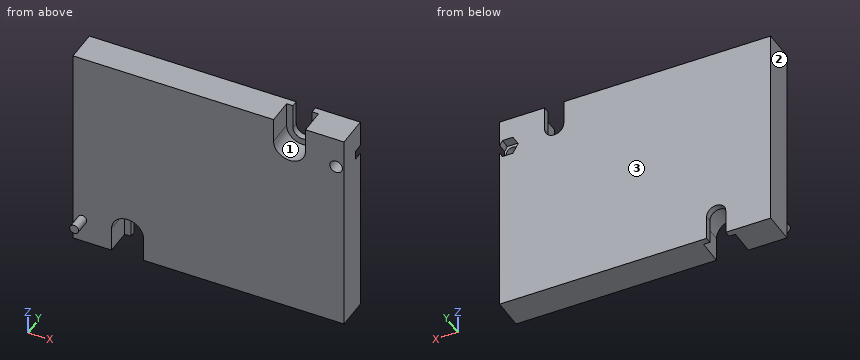
Autodesk Inventor part; units mm, degrees
ref_plane "YZ Plane" through (0, 0, 0) normal (1, 0, 0) x (0, 1, 0)
ref_plane "XZ Plane" through (0, 0, 0) normal (0, 1, 0) x (-1, 0, 0)
ref_plane "XY Plane" through (0, 0, 0) normal (0, 0, 1) x (1, 0, 0)
sketch "Sketch1" plane through (0, 0, 0) normal (0, 1, 0) x (-1, 0, 0)
  line L0 (42.5, -32.5) -> (42.5, 32.5)
  line L1 (-42.5, 32.5) -> (-42.5, -32.5)
  line L2 (-42.5, -32.5) -> (42.5, 32.5) construction
  line L3 (42.5, -32.5) -> (-42.5, 32.5) construction
  line L4 (-25.4, -24.765) -> (25.4, -24.765) construction
  line L5 (25.4, -24.765) -> (25.4, 24.765) construction
  line L6 (25.4, 24.765) -> (-25.4, 24.765) construction
  line L7 (-25.4, 24.765) -> (-25.4, -24.765) construction
  line L8 (-25.4, -24.765) -> (25.4, 24.765) construction
  line L9 (25.4, -24.765) -> (-25.4, 24.765) construction
  arc A0 (-28.4, 24.765) -> (-22.4, 24.765) centre (-25.4, 24.765) ccw
  arc A1 (-30.4, 24.765) -> (-20.4, 24.765) centre (-25.4, 24.765) ccw
  arc A2 (28.4, -24.765) -> (22.4, -24.765) centre (25.4, -24.765) ccw
  arc A3 (30.4, -24.765) -> (20.4, -24.765) centre (25.4, -24.765) ccw
  line L10 (-20.4, 32.5) -> (-20.4, 24.765)
  line L11 (-30.4, 32.5) -> (-30.4, 24.765)
  line L12 (-28.4, 32.5) -> (-28.4, 24.765)
  line L13 (-22.4, 32.5) -> (-22.4, 24.765)
  line L14 (30.4, -24.765) -> (30.4, -32.5)
  line L15 (28.4, -24.765) -> (28.4, -32.5)
  line L16 (22.4, -24.765) -> (22.4, -32.5)
  line L17 (20.4, -24.765) -> (20.4, -32.5)
  line L18 (-42.5, -32.5) -> (22.4, -32.5)
  line L19 (28.4, -32.5) -> (42.5, -32.5)
  line L20 (42.5, 32.5) -> (-22.4, 32.5)
  line L21 (-28.4, 32.5) -> (-42.5, 32.5)
  point P0 (0, 0)
  dimension "d2" = 50.8
  dimension "d3" = 49.53
  dimension "d4" = 6
  dimension "d5" = 10
sketch "Sketch2" plane through (0, 0, 0) normal (0, 1, 0) x (-1, 0, 0)
  line L0 (-43, -29.25) -> (43, -29.25)
  line L1 (43, -29.25) -> (43, 29.25)
  line L2 (43, 29.25) -> (-43, 29.25)
  line L3 (-43, 29.25) -> (-43, -29.25)
  line L4 (-43, -29.25) -> (43, 29.25) construction
  line L5 (43, -29.25) -> (-43, 29.25) construction
  circle A0 centre (39.6, -24.85) radius 1.4
  line L6 (41, -24.85) -> (39.6, -24.85)
  line L7 (39.6, -24.85) -> (39.6, -26.25)
  circle A1 centre (-40, 22.75) radius 2
  line L8 (-38, 22.75) -> (-43, 22.75) construction
  line L9 (-40, 24.75) -> (-40, 29.25) construction
  line L10 (-40, 24.75) -> (-40, 22.75) construction
  point P0 (0, 0)
  dimension "d6" = 86
  dimension "d7" = 58.5
  dimension "d8" = 2.8
  dimension "d9" = 3
  dimension "d10" = 2
  dimension "d11" = 4
  dimension "d12" = 5
  dimension "d13" = 4.5
extrude "Extrusion1" add sketch "Sketch1" along normal blind 10
extrude "Extrusion2" cut sketch "Sketch1" along normal blind 8 contours L19 L15 A2 L16 L18 L17 A3 L14 | L10 A1 L11 L21 L12 A0 L13 L20
extrude "Extrusion3" add sketch "Sketch2" against normal blind 5 contours L6 L7 A0 | A0 L7 L6
extrude "Extrusion4" cut sketch "Sketch2" along normal through all contours A1
sketch "Sketch3" plane through (0, 10, 0) normal (0, 1, 0) x (1, 0, 0)
  circle A0 centre (40, -22.75) radius 2
  arc A1 (-28.4, 24.765) -> (-22.4, 24.765) centre (-25.4, 24.765) ccw
  line L0 (-28.4, 24.765) -> (-28.4, 32.5)
  line L1 (-28.4, 32.5) -> (-42.5, 32.5)
  line L2 (-42.5, 32.5) -> (-42.5, -32.5)
  line L3 (-42.5, -32.5) -> (22.4, -32.5)
  line L4 (22.4, -32.5) -> (22.4, -24.765)
  arc A2 (28.4, -24.765) -> (22.4, -24.765) centre (25.4, -24.765) ccw
  line L5 (28.4, -24.765) -> (28.4, -32.5)
  line L6 (28.4, -32.5) -> (42.5, -32.5)
  line L7 (42.5, -32.5) -> (42.5, 32.5)
  line L8 (42.5, 32.5) -> (-22.4, 32.5)
  line L9 (-22.4, 32.5) -> (-22.4, 24.765)
  circle A3 centre (40, -22.75) radius 2.85
  line L10 (41.6454, -19.9) -> (43.2909, -22.75)
  line L11 (43.2909, -22.75) -> (41.6454, -25.6)
  line L12 (41.6454, -25.6) -> (38.3546, -25.6)
  line L13 (38.3546, -25.6) -> (36.7091, -22.75)
  line L14 (36.7091, -22.75) -> (38.3546, -19.9)
  line L15 (38.3546, -19.9) -> (41.6454, -19.9)
  point P0 (0, 0)
  point P1 (40, -19.9)
  dimension "d22" = 5.7
extrude "Extrusion5" cut sketch "Sketch3" against normal blind 3 contours A0 | A3 L7 | L10 L11 A3 | L7 A3 | A3 L15 L10 | L11 L12 A3 | A3 L14 L15 | L12 L13 A3 | A3 L13 L14
properties part number "base_fuentePoder_12v5a_3DPrint"
Work out the finished part from the listing and answer in its coordinate system (mm). Face numbers are marked on the shaded views. Coordinates: 2 decimals unless noted, no trailing zeros. Write each loop counter-clockwise with the first axis right and the second up, starting at its lowest first coordinate (ties: lowest second). Pieces come first, ordered by that corner, then holes. Notation, with made-up numbers: (79, 54) - (116, 54) arc R20 cw to (116, 87) - close; hole circle Ø2 at (-8, 32). An arc over 180 degrees is marked (long way). One line per question, with ' | ' between items.
1) The mould has two halves that part along X. Classify the marked faces 1, 2 and 3: +X half, -X half, draft (parallel to the pull), parting line (faces both ways), or undercut.
Checks:
face 1: undercut | face 2: -X half | face 3: draft
2) Find section D-D, the plane x = 25.4. Determine the outline of the cut face in (y, z) (3 decimals).
Checks:
outline: (0, -32.5) - (10, -32.5) - (10, 21.765) - (8, 21.765) - (8, 19.765) - (0, 19.765) - close
3) Consider probe 1 along Z at (x, y) = (40, 3.5); probe 2 along Y at (x, z) = (14, -23); probe 3 along X at (y, z) = (4, -27.5). Determine where each line is inside the solid, lowest interval first. Write a range as [from, to].
Checks:
probe 1: [-32.5, 20.75], [24.75, 32.5] | probe 2: [0, 10] | probe 3: [-42.5, -30.4], [-20.4, 42.5]
4) Flat-ended cylindrical pins translate along their axes: P1, Ø2.5, axis at y = 4.5, z = 29, coming from the +X side; P2, Ø3, axis at x = -27, z = -26, coming from the -Y side; P3, Ø8, axis at x = 24, z = 28, coming from the -Y side; P4, Ø4, axis at y = -3, z = 2, coming from the -X side (3 decimals). Find the tip coordinate at first contact, or state that the pin passes through.
Checks:
P1: x = 42.5 | P2: y = 8 | P3: y = 0 | P4: through
5) Find section A-A, the plane y = 1.75. Determine the outline of the cut face in (x, z) (3 decimals).
Checks:
outline: (-42.5, -32.5) - (-30.4, -32.5) - (-30.4, -24.765) arc R5 cw to (-20.4, -24.765) - (-20.4, -32.5) - (42.5, -32.5) - (42.5, 32.5) - (30.4, 32.5) - (30.4, 24.765) arc R5 cw to (20.4, 24.765) - (20.4, 32.5) - (-42.5, 32.5) - close; hole circle Ø4 at (40, 22.75)
6) Find section B-B, the plane x = -39.6. Determine the outline of the cut face in (y, z).
Checks:
outline: (-5, -26.25) - (0, -26.25) - (0, -32.5) - (10, -32.5) - (10, 32.5) - (0, 32.5) - (0, -23.45) - (-5, -23.45) - close
7) Find section C-C, the plane z = -1.5. Determine the outline of the cut face in (x, y), and give its area (3 significant figures).
Checks:
outline: (-42.5, 0) - (42.5, 0) - (42.5, 10) - (-42.5, 10) - close | area: 850 mm2
